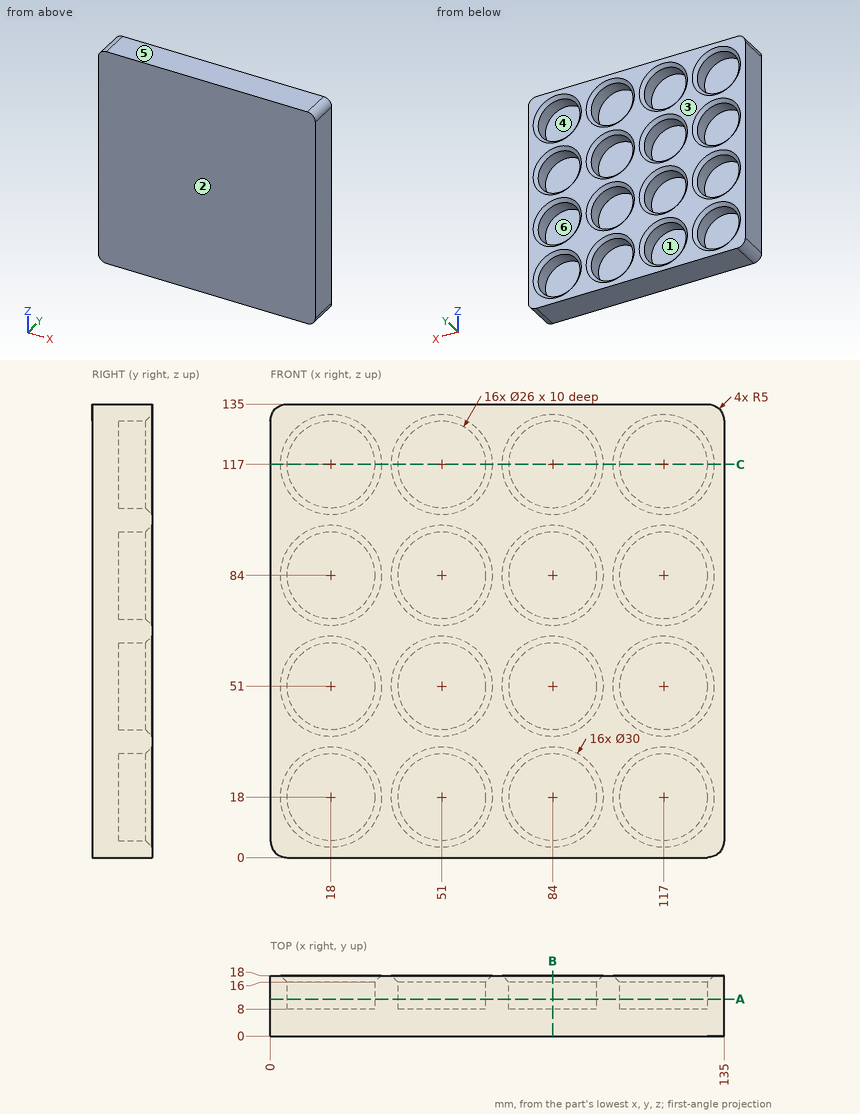
Answer from the drawing. Dimensions are ordinates in mm from the lowest x, y and z of the part. A direction names the side the tool comes from. Coordinates: 2 decimals unless noted, no trailing zeros. Write each loop counter-clockwise with the first axis right and the second up, starting at its lowest first coordinate (ties: lowest second). Pieces come first, ordered by that corner, then holes. Notation, with made-up numbers: M -17.5,12.25 L -9.5,12.25 A25 cw -9.5,40.25 Z; hole C 79.25,-36 d8. An arc over 180 degrees is marked long. Write item = value, one per line.
1. For the marked faces 1 and 2, determine the directions among +Z, -Z, +X, -X, +Y, -Y from which every point of the face is accessible in a straight line to the end or side of a thin tool.
Solution:
face_1 = +Y
face_2 = +Z, -Z, +X, -X, -Y
2. The part is cut by section B-B (x = 84). Determine the outline of the cut face in (y, z).
Solution:
outline = M 0,0 L 18,0 L 18,3 L 16,5 L 8,5 L 8,31 L 16,31 L 18,33 L 18,36 L 16,38 L 8,38 L 8,64 L 16,64 L 18,66 L 18,69 L 16,71 L 8,71 L 8,97 L 16,97 L 18,99 L 18,102 L 16,104 L 8,104 L 8,130 L 16,130 L 18,132 L 18,135 L 0,135 Z
3. The part is cut by section C-C (z = 117). Determine the outline of the cut face in (x, y).
Solution:
outline = M 0,0 L 135,0 L 135,18 L 132,18 L 130,16 L 130,8 L 104,8 L 104,16 L 102,18 L 99,18 L 97,16 L 97,8 L 71,8 L 71,16 L 69,18 L 66,18 L 64,16 L 64,8 L 38,8 L 38,16 L 36,18 L 33,18 L 31,16 L 31,8 L 5,8 L 5,16 L 3,18 L 0,18 Z
4. The part is cut by section A-A (y = 11). State how many separate pieces and enclosed holes the cut face has, then the cut area to 3 significant figures.
Solution:
separate_pieces = 1
enclosed_holes = 16
area = 9,710 mm2
5. Straight lines are drawn through the part: line 1 (X direction, y = 14.5, z = 84); line 2 (X direction, y = 12.5, z = 74). For each, find the intervals that lie inside material, in ascending order. Write a range as from..to.
Solution:
line_1 = 0..5, 31..38, 64..71, 97..104, 130..135
line_2 = 0..9.69, 26.31..42.69, 59.31..75.69, 92.31..108.69, 125.31..135
6. A flat-ended cylindrical pin translates along its axis: pin 1 (15.5 mm diameter, centred on x = 18, z = 51, fed in from +Y). Find the tip coordinate at first contact, or state that the pin passes through.
Solution:
pin_1 = 8
7. Determine the mould class of the marked faces 3, 4, 5 and 6 for opening direction Z: released by +Z, released by -Z, zero draft, split by the parting line, or undercut.
Solution:
face_3 = zero draft
face_4 = undercut
face_5 = released by +Z
face_6 = undercut
